Design review of the part shown in the three views and the two pictorial views. Dimensions are in mm from the part's minimum x, y and z. Coordinates: 2 decimals unless noted, no trailing zeros. Loops run counter-clockwise (first coordinate to the right, second up) from the corner with the lowest first, then second, coordinate; pieces in that order, holes last. Notation, with made-up numbers: M -12,-8.75 L 47,-8.75 A10 ccw 47,4.25 Z; hole C 9,81 d8. An arc over 180 degrees is marked long. Answer as a JSON object with one key per item and string values. Group by question number.
Item 1: Add section C-C (y = 88.1). State the section outline as (x, z) points, then the cut area to 3 significant figures.
Item 2: Add section B-B (z = 1.25). State the section outline as (x, y) points.
Item 3: Wall thickness on L1, parallel to X at y = 88.1, z = 4.5; L2, parallel to Y at x = 40, z = 5.5; L3, parallel to X at y = 88.5, z = 1: over which ranges is each line inside the solid? List them lowest first. Write a range as from..to.
Item 4: Insertion check: pin 1 (7 mm diameter, centred on x = 40, y = 88.1, fed in from -Z); pin 2 (6.5 mm diameter, centred on x = 10, y = 88.1, fed in from -Z). Each pin has a flat end and moves straight along its axis. Give the tip position at first contact, or say it passes through.
Item 5: Add section A-A (x = 10). State the section outline as (y, z) points, then the cut area to 3 significant figures.
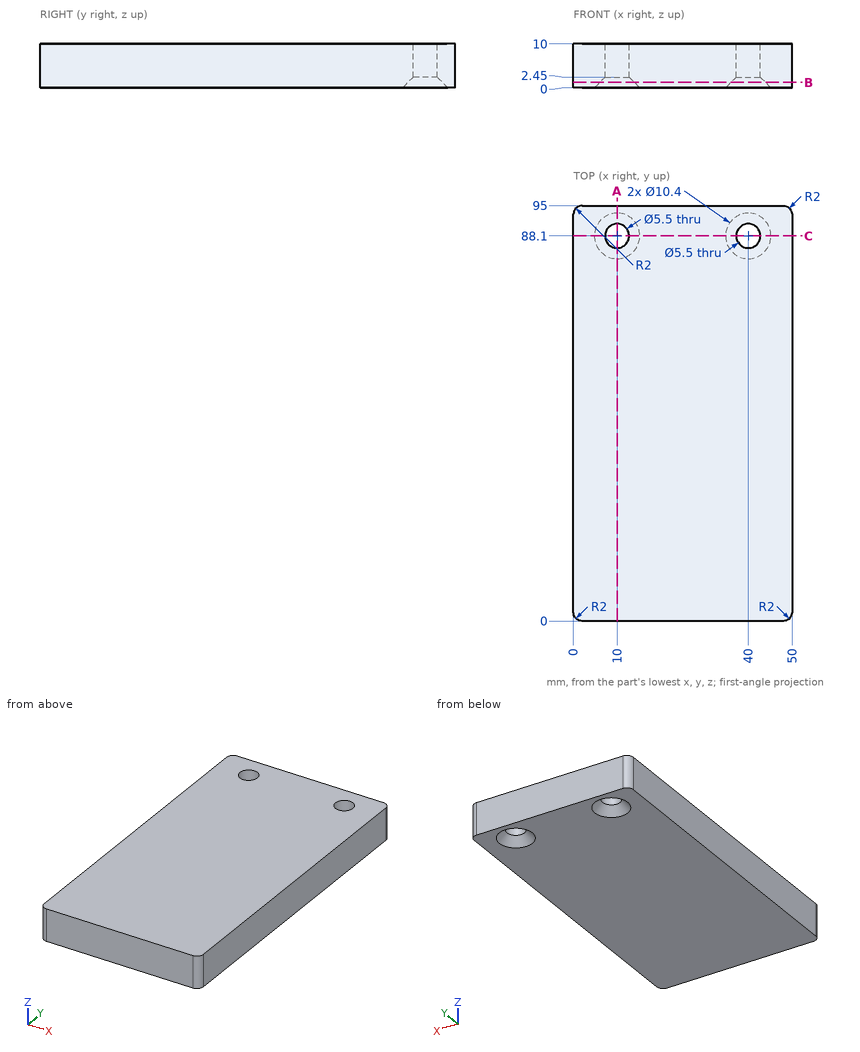
From the geometry:
{
 "1": {"outline": "M 0,0 L 4.8,0 L 7.25,2.45 L 7.25,10 L 0,10 Z; M 12.75,2.45 L 15.2,0 L 34.8,0 L 37.25,2.45 L 37.25,10 L 12.75,10 Z; M 42.75,2.45 L 45.2,0 L 50,0 L 50,10 L 42.75,10 Z", "area": "378 mm²"},
 "2": {"outline": "M 0,2 A2 ccw 2,0 L 48,0 A2 ccw 50,2 L 50,93 A2 ccw 48,95 L 2,95 A2 ccw 0,93 Z; hole C 10,88.1 d7.9; hole C 40,88.1 d7.9"},
 "3": {"L1": "x = 0..7.25, 12.75..37.25, 42.75..50", "L2": "y = 0..85.35, 90.85..95", "L3": "x = 0..5.82, 14.18..35.82, 44.18..50"},
 "4": {"pin 1": "stops at z = 1.7", "pin 2": "stops at z = 1.95"},
 "5": {"outline": "M 0,0 L 82.9,0 L 85.35,2.45 L 85.35,10 L 0,10 Z; M 90.85,2.45 L 93.3,0 L 95,0 L 95,10 L 90.85,10 Z", "area": "889 mm²"}
}
